Source: three-view drawing plus pictorial views. Frame: mm from the lowest corner of the part. Coordinates: 2 decimals unless noted, no trailing zeros. Loops run counter-clockwise (first coordinate to the right, second up) from the corner with the lowest first, then second, coordinate; pieces in that order, holes last. Notation, with made-up numbers: M 70.25,7 L 117.25,7 A18 cw 117.25,40 Z; hole C 76.5,48 d4. An arc over 180 degrees is marked long. Write each question's results on one line, items separated by ' | '. Start each with the question number.
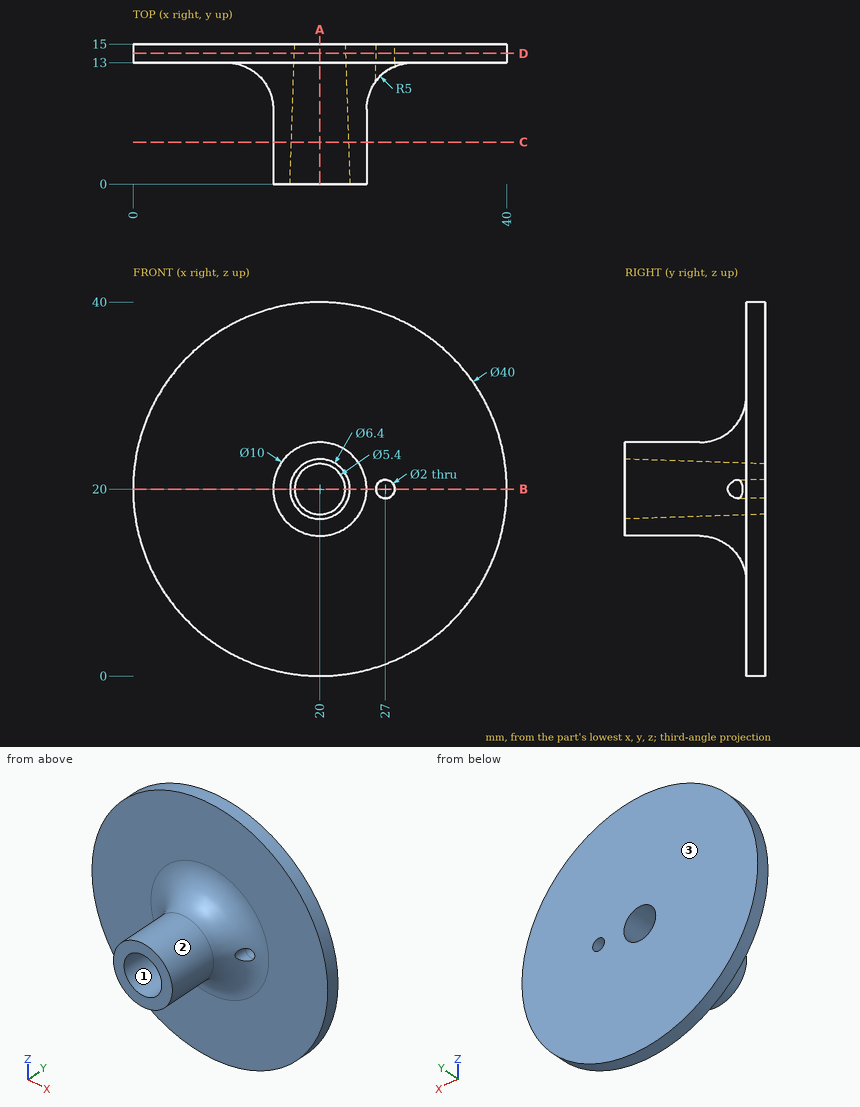
Item 1: Section C-C, the plane y = 4.5. Return loops of the section in (x, z), plus the area to 3 significant figures.
Item 2: Ray query, L1, parallel to Y at x = 30, z = 35; L2, parallel to X at y = 4.75, z = 17.5; L3, parallel to X at y = 12.05, z = 20. Return the intervals inside material, ascending. Write a range as [from, to].
Item 3: Contact query for flat-ended pins moving along their axis: P1, Ø3, axis at x = 27, z = 20, coming from the -Y side; P2, Ø4, axis at x = 19, y = 2.5, coming from the -Z side; P3, Ø1.5, axis at y = 8.5, z = 17, coming from the +X side. Output: stop coordinate, or through.
Item 4: Section D-D, the plane y = 14. Return loops of the section in (x, z).
Item 5: Section B-B, the plane z = 20. Return loops of the section in (x, y), plus the area to 3 significant figures.
Item 6: Section A-A, the plane x = 20. Return loops of the section in (y, z), plus the area to 3 significant figures.
Item 7: Pull-direction query (X, two-part tool) for the marked faces 1, 2 and 3; classes: released by +X, released by -X, zero draft, split by the parting line, or undercut.
Solutions:
1) outline: C 20,20 d10; hole C 20,20 d6.1 | area: 49.3 mm²
2) L1: y = [13, 15] | L2: x = [15.67, 18.27], [21.73, 24.33] | L3: x = [12.93, 17.2], [22.8, 26]
3) P1: stops at y = 10.18 | P2: stops at z = 15 | P3: stops at x = 24.51
4) outline: C 20,20 d40; hole C 20,20 d5.47; hole C 27,20 d2
5) outline: M 0,13 L 10,13 A5 cw 15,8 L 15,0 L 16.8,0 L 17.3,15 L 0,15 Z; M 22.7,15 L 23.2,0 L 25,0 L 25,8 A5 cw 26,11 L 26,15 Z; M 28,12.58 A5 cw 30,13 L 40,13 L 40,15 L 28,15 Z | area: 126 mm²
6) outline: M 0,15 L 8,15 A5 cw 13,10 L 13,0 L 15,0 L 15,17.3 L 0,16.8 Z; M 0,23.2 L 15,22.7 L 15,40 L 13,40 L 13,30 A5 cw 8,25 L 0,25 Z | area: 132 mm²
7) face 1: undercut | face 2: split by the parting line | face 3: zero draft
